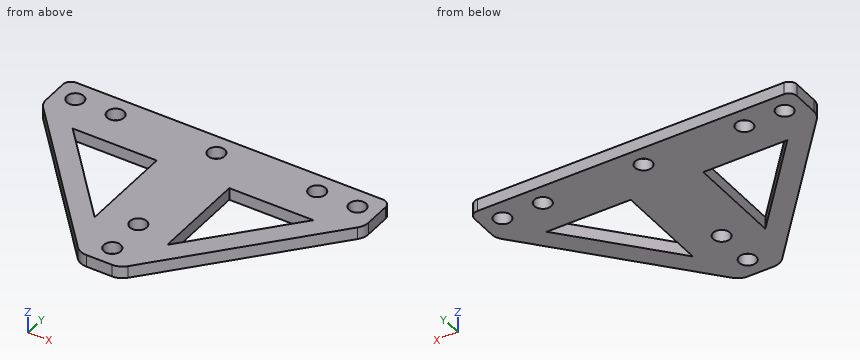
```python
from build123d import *

# Parameters (mm, degrees)
EXTRUDE_1_DEPTH     = 3
SKETCH_2_R          = 2.1
CUT_EXTRUDE_1_DEPTH = 95.387499172
CUT_EXTRUDE_2_DEPTH = 95.387499172
FILLET_1_R          = 2
FILLET_2_R          = 4


with BuildPart() as part:
    # 草图1 → 凸台-拉伸1 (new body)
    with BuildSketch(Plane.XY):
        Polygon((0, 0), (80, 0), (80, -10), (45, -50), (35, -50), (0, -10), align=None)
    extrude(amount=EXTRUDE_1_DEPTH)

    # 草图2 → 切除-拉伸1 (cut, through all)
    with BuildSketch(Plane.XY.offset(3)):
        with Locations((5, -5)):
            Circle(SKETCH_2_R)
        with Locations((15, -5)):
            Circle(SKETCH_2_R)
        with Locations(Location((65, -5, 0), (0, 0, 180))):
            Circle(SKETCH_2_R)
        with Locations(Location((75, -5, 0), (0, 0, 180))):
            Circle(SKETCH_2_R)
        with Locations((40, -45)):
            Circle(SKETCH_2_R)
        with Locations((40, -35)):
            Circle(SKETCH_2_R)
        with Locations((40, -5)):
            Circle(SKETCH_2_R)
    extrude(amount=-CUT_EXTRUDE_1_DEPTH, mode=Mode.SUBTRACT)

    # 草图3 → 切除-拉伸2 (cut, through all)
    with BuildSketch(Plane.XY.offset(3)):
        Polygon((10.143841133, -14), (31, -14), (31, -37.835610134), align=None)
        Polygon((49, -37.835610134), (69.856158867, -14), (49, -14), align=None)
    extrude(amount=-CUT_EXTRUDE_2_DEPTH, mode=Mode.SUBTRACT)

    # 圆角1
    fillet_1_edges = [part.edges().sort_by_distance(p)[0] for p in [
        (0, 0, 1.5),
        (80, 0, 1.5),
    ]]
    fillet(fillet_1_edges, radius=FILLET_1_R)

    # 圆角2
    fillet_2_edges = [part.edges().sort_by_distance(p)[0] for p in [
        (80, -10, 1.5),
        (45, -50, 1.5),
        (35, -50, 1.5),
        (0, -10, 1.5),
    ]]
    fillet(fillet_2_edges, radius=FILLET_2_R)


solid = part.part
```
Geometry check sheet. Reference: the model listing, model coordinates, mm. Round coordinates to 2 decimals unless told otherwise and drop trailing zeros. Loops run counter-clockwise (first coordinate to the right, second up) from the corner with the lowest first, then second, coordinate; pieces in that order, holes last. Notation, with made-up numbers: (11.5, 80) - (21.5, 80) arc R21 cw to (21.5, 115) - close; hole circle Ø3 at (-8, 69). An arc over 180 degrees is marked (long way). Write item = value, one per line. Start each with the question number.
1. Thickness scan on line 1 (Y direction, x = 40, z = 1.35); line 2 (X direction, y = -17.5, z = 1.65); line 3 (Y direction, x = 65, z = 0.9). Record the ranges inside material, lowest first.
2. Section check D-D on y = -18. Enter the section's corners in (x, z).
3. Section check C-C on x = 40. Enter the section's corners in (y, z).
4. Depth check by flat-ended pin: pin 1 (5.5 mm diameter, centred on x = 75, y = -5, fed in from -Z); pin 2 (1.5 mm diameter, centred on x = 64.5, z = 1.5, fed in from -Y); pin 3 (1.5 mm diameter, centred on y = -42, z = 2.5, fed in from +X); pin 4 (0.9 mm diameter, centred on x = 23, z = 1.5, fed in from -Y). Enter the tip coordinate at first touch or a pass-through.
5. Section check A-A on y = -5. Enter the section's corners in (x, z), then the cut area to 3 significant figures.
6. Section check B-B on z = 1.55. Give the number of separate pieces and of enclosed holes in the cut face, then the cut area to 3 significant figures.
Working result:
q1.line_1 = -50 to -47.1, -42.9 to -37.1, -32.9 to -7.1, -2.9 to 0
q1.line_2 = 6.56 to 13.21, 31 to 49, 66.79 to 73.44
q1.line_3 = -27.14 to -19.55, -14 to -7.1, -2.9 to 0
q2.outline = (7, 0) - (13.64, 0) - (13.64, 3) - (7, 3) - close; (31, 0) - (49, 0) - (49, 3) - (31, 3) - close; (66.36, 0) - (73, 0) - (73, 3) - (66.36, 3) - close
q3.outline = (-50, 0) - (-47.1, 0) - (-47.1, 3) - (-50, 3) - close; (-42.9, 0) - (-37.1, 0) - (-37.1, 3) - (-42.9, 3) - close; (-32.9, 0) - (-7.1, 0) - (-7.1, 3) - (-32.9, 3) - close; (-2.9, 0) - (0, 0) - (0, 3) - (-2.9, 3) - close
q4.pin_1 = 0
q4.pin_2 = -28.57
q4.pin_3 = 52.66
q4.pin_4 = -36.8
q5.outline = (0, 0) - (2.9, 0) - (2.9, 3) - (0, 3) - close; (7.1, 0) - (12.9, 0) - (12.9, 3) - (7.1, 3) - close; (17.1, 0) - (37.9, 0) - (37.9, 3) - (17.1, 3) - close; (42.1, 0) - (62.9, 0) - (62.9, 3) - (42.1, 3) - close; (67.1, 0) - (72.9, 0) - (72.9, 3) - (67.1, 3) - close; (77.1, 0) - (80, 0) - (80, 3) - (77.1, 3) - close
q5.area = 177 mm^2
q6.separate_pieces = 1
q6.enclosed_holes = 9
q6.area = 2,000 mm^2
